For this review, use the dimensioned drawing (mm, ordinates from the lowest corner) and the shaded views. A direction names the side the tool comes from. Coordinates: 2 decimals unless noted, no trailing zeros. Loops run counter-clockwise (first coordinate to the right, second up) from the corner with the lowest first, then second, coordinate; pieces in that order, holes last. Notation, with made-up numbers: (61.25, 5.5) -> (106.25, 5.5) arc R22 ccw to (106.25, 13.5) -> close; hole circle Ø6 at (-19, 39.25). An arc over 180 degrees is marked (long way). Answer as a JSON object with one key per item and string values.
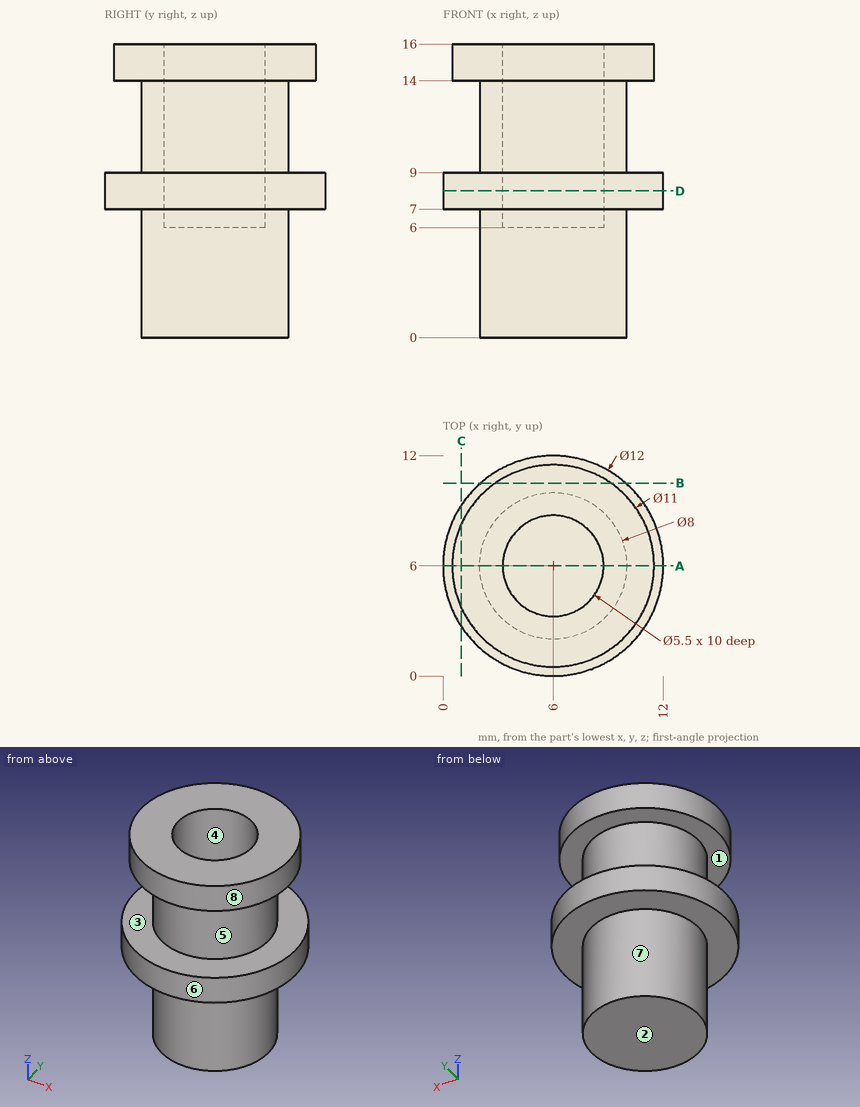
1) The part is to be moulded in two halves that separate along Z. For the marked faces 1, 2, 3 and 4, say which applies: pulls with the +Z half, pulls with the -Z half, needs draft (parallel to the pull), parting line crosses it, or undercut.
Completed:
{"face 1": "undercut", "face 2": "pulls with the -Z half", "face 3": "undercut", "face 4": "needs draft"}
2) For the marked faces 5, 6, 7 and 8, list the 3-axis set-ups (+Z, -Z, +X, -X, +Y, -Y) from which the entire face can be reached by the end or side of a thin tool; tool diameter is ignored.
Completed:
{"face 5": "none", "face 6": "+Z, -Z", "face 7": "-Z", "face 8": "+Z"}
3) Add section C-C, the plane x = 1. Give the boundary of the cut face in (y, z).
Completed:
{"outline": "(2.68, 7) -> (9.32, 7) -> (9.32, 9) -> (2.68, 9) -> close; (3.71, 14) -> (8.29, 14) -> (8.29, 16) -> (3.71, 16) -> close"}
4) Clearance check with a flat-ended pin moving along its axis: pin 1 Ø3 at (x, z) = (9.5, 11) entering from +Y. State where the tip first meets the part, or that it passes through.
Completed:
{"pin 1": "y = 9.46"}
5) Add section A-A, the plane y = 6. Give the boundary of the cut face in (x, z).
Completed:
{"outline": "(0, 7) -> (2, 7) -> (2, 0) -> (10, 0) -> (10, 7) -> (12, 7) -> (12, 9) -> (10, 9) -> (10, 14) -> (11.5, 14) -> (11.5, 16) -> (8.75, 16) -> (8.75, 6) -> (3.25, 6) -> (3.25, 16) -> (0.5, 16) -> (0.5, 14) -> (2, 14) -> (2, 9) -> (0, 9) -> close"}
6) Add section D-D, the plane z = 8. Give the boundary of the cut face in (x, y).
Completed:
{"outline": "circle Ø12 at (6, 6); hole circle Ø5.5 at (6, 6)"}
7) Add section B-B, the plane y = 10.5. Give the boundary of the cut face in (x, z).
Completed:
{"outline": "(2.03, 7) -> (9.97, 7) -> (9.97, 9) -> (2.03, 9) -> close; (2.84, 14) -> (9.16, 14) -> (9.16, 16) -> (2.84, 16) -> close"}
8) Wall thickness on probe 1 along Y at (x, z) = (6, 9.25); probe 2 along Z at (x, y) = (10.25, 2.75); probe 3 along Y at (x, z) = (6, 8.75): over which ranges is each line inside the solid? List them lowest first.
Completed:
{"probe 1": "2 to 3.25, 8.75 to 10", "probe 2": "7 to 9, 14 to 16", "probe 3": "0 to 3.25, 8.75 to 12"}
